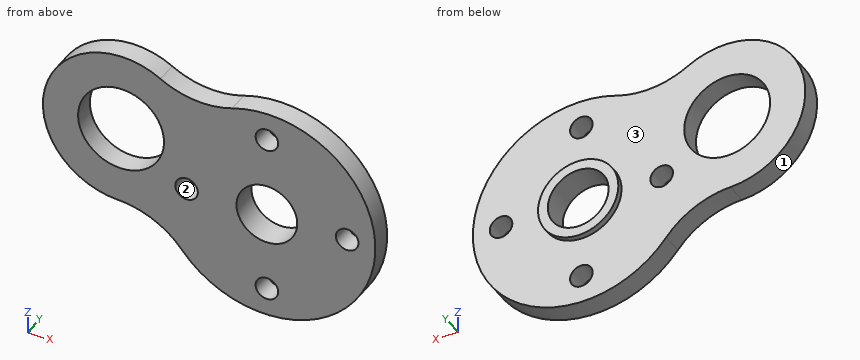
```python
from build123d import *

# Parameters (mm, degrees)
SKETCH2_R           = 25
SKETCH2_R_2         = 2.6
BOSS_EXTRUDE1_DEPTH = 5
SKETCH4_R           = 9.25
BOSS_EXTRUDE2_DEPTH = 1.35
SKETCH3_R           = 7
CUT_EXTRUDE1_DEPTH  = 36.921059283
SKETCH5_R           = 9.9
BOSS_EXTRUDE3_DEPTH = 5
FILLET1_R           = 20


with BuildPart() as part:
    # Sketch2 → Boss-Extrude1 (new body)
    with BuildSketch(Plane(origin=(0, 0, 0), x_dir=(1, 0, 0), z_dir=(0, 1, 0))):
        with Locations(Location((0, 0, 0), (0, 0, 270))):
            Circle(SKETCH2_R)
        with Locations(Location((0, 18.5, 0), (0, 0, 270))):
            Circle(SKETCH2_R_2, mode=Mode.SUBTRACT)
        with Locations(Location((18.5, 0, 0), (0, 0, 270))):
            Circle(SKETCH2_R_2, mode=Mode.SUBTRACT)
        with Locations(Location((0, -18.5, 0), (0, 0, 270))):
            Circle(SKETCH2_R_2, mode=Mode.SUBTRACT)
        with Locations(Location((-18.5, 0, 0), (0, 0, 270))):
            Circle(SKETCH2_R_2, mode=Mode.SUBTRACT)
    extrude(amount=BOSS_EXTRUDE1_DEPTH)

    # Sketch4 → Boss-Extrude2 (add)
    with BuildSketch(Plane(origin=(0, 5, 0), x_dir=(1, 0, 0), z_dir=(0, 1, 0))):
        with Locations(Location((0, 0, 0), (0, 0, 90))):
            Circle(SKETCH4_R)
    extrude(amount=BOSS_EXTRUDE2_DEPTH)

    # Sketch3 → Cut-Extrude1 (cut, through all)
    with BuildSketch(Plane(origin=(0, 6.35, 0), x_dir=(1, 0, 0), z_dir=(0, 1, 0))):
        with Locations(Location((0, 0, 0), (0, 0, 270))):
            Circle(SKETCH3_R)
    extrude(amount=-CUT_EXTRUDE1_DEPTH, mode=Mode.SUBTRACT)

    # Sketch5 → Boss-Extrude3 (add)
    with BuildSketch(Plane.XZ):
        with BuildLine():
            ThreePointArc((-17.474868047, 17.878170677), (-50.857855513, 14.915714286), (-24.362914979, -5.607884962))
            ThreePointArc((-24.362914979, -5.607884962), (-23.989554487, 7.035714286), (-17.474868047, 17.878170677))
        make_face()
        with Locations(Location((-33.585376282, 9.85, 0), (0, 0, 270))):
            Circle(SKETCH5_R, mode=Mode.SUBTRACT)
    extrude(amount=-BOSS_EXTRUDE3_DEPTH)

    # Fillet1
    fillet1_edges = [part.edges().sort_by_distance(p)[0] for p in [
        (-17.474868047, 2.5, 17.878170677),
        (-24.362914979, 2.5, -5.607884962),
    ]]
    fillet(fillet1_edges, radius=FILLET1_R)


solid = part.part
```
CAD build for the part. Positions are in the model's coordinates, mm. Face numbers are marked on the shaded views. Coordinates: 2 decimals unless noted, no trailing zeros. Write each loop counter-clockwise with the first axis right and the second up, starting at its lowest first coordinate (ties: lowest second). Pieces come first, ordered by that corner, then holes. Notation, with made-up numbers: (69, 85) -> (97, 85) arc R11 cw to (97, 89) -> close; hole circle Ø6 at (-39.5, -13). An arc over 180 degrees is marked (long way). Return JSON: item names as keys, results as strings. Group by question number.
Q1. Cut at B-B, the plane z = -20. Give the cut face in (x, y), then the cut area to 3 significant figures.
Q2. Flat gauge pins, fed straight in: pin 1 (3 mm diameter, centred on x = -18.5, y = 3.5, fed in from -Z); pin 2 (16 mm diameter, centred on x = -23, z = 13, fed in from +Y); pin 3 (4.5 mm diameter, centred on x = 0, z = -18.5, fed in from +Y); pin 4 (1.5 mm diameter, centred on y = 1, z = 8, fed in from +X). Where does each tip first touch, or does it go through?
Q3. Pull direction X, two halves, no side cores. Call the marked faces 1, 2 and 3: released by +X, released by -X, zero draft, split by the parting line, or undercut.
Q4. Drill centre lines: line 1 (X direction, y = 2.25, z = 18.5); line 2 (X direction, y = 0.75, z = 3); line 3 (Y direction, x = -10.5, z = 9.5). Where is each one in solid material? Low to high.
Q5. Cut at A-A, the plane x = 0. Give the cut face in (y, z), then the cut area to 3 significant figures.
Q6. Cut at C-C, the plane z = 18.5. Give the cut face in (x, y).
Q7. Cut at D-D, the plane x = -39.5. Give the cut face in (y, z).
Returned:
{
 "1": {"outline": "(-15, 0) -> (-2.12, 0) -> (-2.12, 5) -> (-15, 5) -> close; (2.12, 0) -> (15, 0) -> (15, 5) -> (2.12, 5) -> close", "area": "129 mm2"},
 "2": {"pin 1": "stops at z = -18.33", "pin 2": "stops at y = 5", "pin 3": "passes through", "pin 4": "stops at x = 23.93"},
 "3": {"face 1": "split by the parting line", "face 2": "undercut", "face 3": "zero draft"},
 "4": {"line 1": "x = -49.37 to -38.4, -28.77 to -2.6, 2.6 to 16.82", "line 2": "x = -50.23 to -40.73, -26.44 to -6.32, 6.32 to 24.82", "line 3": "y = 0 to 5"},
 "5": {"outline": "(0, -25) -> (5, -25) -> (5, -21.1) -> (0, -21.1) -> close; (0, -15.9) -> (5, -15.9) -> (5, -9.25) -> (6.35, -9.25) -> (6.35, -7) -> (0, -7) -> close; (0, 7) -> (6.35, 7) -> (6.35, 9.25) -> (5, 9.25) -> (5, 15.9) -> (0, 15.9) -> close; (0, 21.1) -> (5, 21.1) -> (5, 25) -> (0, 25) -> close", "area": "134 mm2"},
 "6": {"outline": "(-49.37, 0) -> (-38.4, 0) -> (-38.4, 5) -> (-49.37, 5) -> close; (-28.77, 0) -> (-2.6, 0) -> (-2.6, 5) -> (-28.77, 5) -> close; (2.6, 0) -> (16.82, 0) -> (16.82, 5) -> (2.6, 5) -> close"},
 "7": {"outline": "(0, -7.15) -> (5, -7.15) -> (5, 1.91) -> (0, 1.91) -> close; (0, 17.79) -> (5, 17.79) -> (5, 26.85) -> (0, 26.85) -> close"}
}
